Read the model definition and answer for the solid it produces. Units are mm, in the model's axes. Round coordinates to 2 decimals unless told otherwise and drop trailing zeros. Order: outer loops, then holes, each group sorted by start corner. A loop starts at its lowest first (then second) coordinate and runs counter-clockwise, first axis right, second up. Notation, with made-up numbers: (-4.5, 11) - (52.5, 11) arc R12 cw to (52.5, 29) - close; hole circle Ø11 at (86.25, -7.75). An arc over 180 degrees is marked (long way). Put each result on its own line as item: value. Start each with the question number.
Q1. Section C-C on z = 12.25 is taken. Give the vertices of the cut face in (x, y), then the cut area to 3 significant figures.
Q2. This flat-tipped pin is pushed along its axis until it touches: pin 1 Ø5 at (x, z) = (5, 12.5) entering from -Y. Where does it stop, or does it pass through?
Q3. For a pull along Z with two mould halves and no side action, classify faces 1 (the face through (16.17, -69.84, 12.52)), 2 (the face through (16, 0, 7)), 3 (the face through (16, -32, 0)) as pulls with the +Z half, pulls with the -Z half, needs draft (parallel to the pull), parting line crosses it, or undercut.
Q4. Find the intervals of material crossed by line 1 along Y through (x, z) = (27, 4.5); line 2 along Y through (x, z) = (29, 2.75), in increasing order. Write a range as from..to.
Q5. Section A-A on x = 8 is taken. Give the vertices of the cut face in (y, z) (3 decimals), then the cut area to 3 significant figures.
Q6. Section B-B on z = 3.25 is taken. Give the vertices of the cut face in (x, y).
from build123d import *

# Parameters (mm, degrees)
F0_W        = 32.8
F0_H        = 14.57
F1_DEPTH    = 72.34
F2_T1_DEPTH = 71.55
F3_R        = 1


# Not quite as in the source:
# - a fillet or chamfer that OpenCascade refuses, or shapes differently, is made with other operations: its cross-section is extruded or revolved along the edge and cut away or added


with BuildPart() as f1:
    # F0 (on Front) → F1 (new body)
    with BuildSketch(Plane.XZ):
        with Locations((16.4, 7.285)):
            Rectangle(F0_W, F0_H)
    extrude(amount=F1_DEPTH)

    # F2: fillet of radius 7.75 on 2 edges, made by hand

    # F2_s2 → F2_t1 (cut)
    with BuildSketch(Plane.YZ.offset(-19.375)):
        with BuildLine():
            ThreePointArc((-64.59, 14.57), (-70.0700775542, 12.3000775542), (-72.34, 6.82))
            Line((-72.34, 6.82), (-72.34, 14.57))
            Line((-72.34, 14.57), (-64.59, 14.57))
        make_face()
        with BuildLine():
            ThreePointArc((-64.59, 0), (-70.0700775542, 2.2699224458), (-72.34, 7.75))
            Line((-72.34, 7.75), (-72.34, 0))
            Line((-72.34, 0), (-64.59, 0))
        make_face()
    extrude(amount=F2_T1_DEPTH, mode=Mode.SUBTRACT)

    # F3
    f3_edges = [f1.edges().sort_by_distance(p)[0] for p in [
        (0, 0, 7.285),
        (32.8, 0, 7.285),
    ]]
    fillet(f3_edges, radius=F3_R)


solid = f1.part
Findings:
1. outline: (0, -70.12) - (32.8, -70.12) - (32.8, -1) arc R1 ccw to (31.8, 0) - (1, 0) arc R1 ccw to (0, -1) - close
1. area: 2,300 mm2
2. pin 1: y = -71.66
3. face 1: pulls with the +Z half
3. face 2: needs draft
3. face 3: pulls with the -Z half
4. line 1: -71.63..0
4. line 2: -70.51..0
5. outline: (-72.326, 7.285) arc R7.75 ccw to (-64.59, 0) - (0, 0) - (0, 14.57) - (-64.59, 14.57) arc R7.75 ccw to start
5. area: 1,030 mm2
6. outline: (0, -70.9) - (32.8, -70.9) - (32.8, -1) arc R1 ccw to (31.8, 0) - (1, 0) arc R1 ccw to (0, -1) - close
